from build123d import *

# Parameters (mm, degrees)
EXTRUDE_1_DEPTH = 5.5
SKETCH_2_W      = 7.3
SKETCH_2_H      = 7.8
EXTRUDE_2_DEPTH = 2.7
FILLET_1_R      = 1
CHAMFER_1_SIZE  = 1


with BuildPart() as part:
    # Эскиз1 → Бобышка-Вытянуть1 (new body)
    with BuildSketch(Plane.XY):
        with BuildLine():
            Line((0, 2.4), (7.5, 2.4))
            ThreePointArc((7.5, 2.4), (9.9, 0), (7.5, -2.4))
            Line((7.5, -2.4), (0, -2.4))
            ThreePointArc((0, -2.4), (-2.4, 0), (0, 2.4))
        make_face()
    extrude(amount=EXTRUDE_1_DEPTH)

    # Эскиз2 → Бобышка-Вытянуть2 (add)
    with BuildSketch(Plane.XY.offset(5.5)):
        with Locations((3.75, 0)):
            Rectangle(SKETCH_2_W, SKETCH_2_H)
    extrude(amount=-EXTRUDE_2_DEPTH)

    # Скругление1
    fillet_1_edges = [part.edges().sort_by_distance(p)[0] for p in [
        (3.75, 2.4, 0),
        (9.9, 0, 0),
        (3.75, -2.4, 0),
        (-2.4, 0, 0),
    ]]
    fillet(fillet_1_edges, radius=FILLET_1_R)

    # Фаска1
    chamfer_1_edges = [part.edges().sort_by_distance(p)[0] for p in [
        (3.75, -3.9, 5.5),
        (3.75, 3.9, 5.5),
    ]]
    chamfer(chamfer_1_edges, length=CHAMFER_1_SIZE)


solid = part.part
The listing builds one solid part. Answer for the finished solid, in the listing's coordinates (mm). A direction names the side the tool comes from. Coordinates: 2 decimals unless noted, no trailing zeros. Loops run counter-clockwise (first coordinate to the right, second up) from the corner with the lowest first, then second, coordinate; pieces in that order, holes last.
1) Find the intervals of material crossed by L1, parallel to Y at x = 0, z = 2.6; L2, parallel to X at y = 3.5, z = 3.7; L3, parallel to X at y = 2, z = 1.75, in increasing order.
2) Find section A-A on x = 2. Write down the section's boundary in (y, z).
3) Find section B-B on z = 4.65. Write down the section's boundary in (x, y), then the cut area to 3 significant figures.
4) Find section D-D on z = 1.95. Write down the section's boundary in (x, y), then the cut area to 3 significant figures.
5) A tool of negligible diameter and unlimited length cuts with its end or side. For faces 1 (the face through (4, -3, 2.8)), 2 (the face through (0.1, -3, 4)), 3 (the face through (0.1, 3, 4)), from which of +Z, -Z, +X, -X, +Y, -Y can it reach the whole face along a straight path? Write none if from no direction.
6) Flat-ended cylindrical pins translate along their axes: pin 1 Ø0.8 at (y, z) = (3, 4.5) entering from +X; pin 2 Ø2 at (x, z) = (4, 1.5) entering from -Y; pin 3 Ø0.8 at (y, z) = (-3.5, 4.5) entering from -X. Find the tip coordinate at first contact, or state that the pin passes through.
7) Find section C-C on y = 2.75. Write down the section's boundary in (x, z).
Values:
1. L1: y = -2.4 to 2.4
1. L2: x = 0.1 to 7.4
1. L3: x = -1.33 to 8.83
2. outline: (-3.9, 2.8) - (-2.4, 2.8) - (-2.4, 1) arc R1 ccw to (-1.4, 0) - (1.4, 0) arc R1 ccw to (2.4, 1) - (2.4, 2.8) - (3.9, 2.8) - (3.9, 4.5) - (2.9, 5.5) - (-2.9, 5.5) - (-3.9, 4.5) - close
3. outline: (0, -2.4) - (0.1, -2.4) - (0.1, -3.75) - (7.4, -3.75) - (7.4, -2.4) - (7.5, -2.4) arc R2.4 ccw to (7.5, 2.4) - (7.4, 2.4) - (7.4, 3.75) - (0.1, 3.75) - (0.1, 2.4) - (0, 2.4) arc R2.4 ccw to start
3. area: 73.8 mm2
4. outline: (0, -2.4) - (7.5, -2.4) arc R2.4 ccw to (7.5, 2.4) - (0, 2.4) arc R2.4 ccw to start
4. area: 54.1 mm2
5. face 1: -Z, +X, -X, -Y
5. face 2: +Z, -Z, -X, -Y
5. face 3: +Z, -Z, -X, +Y
6. pin 1: stops at x = 7.4
6. pin 2: stops at y = -2.4
6. pin 3: stops at x = 0.1
7. outline: (0.1, 2.8) - (7.4, 2.8) - (7.4, 5.5) - (0.1, 5.5) - close
